Read the model definition and answer for the solid it produces. Units are mm, in the model's axes. A direction names the side the tool comes from. Give positions to 0.01 mm unless a question says otherwise; leave off trailing zeros. Write each loop counter-clockwise with the first axis right and the second up, starting at its lowest first coordinate (ties: lowest second). Pieces come first, ordered by that corner, then holes. Notation, with made-up numbers: M 50.25,32.25 L 87.25,32.25 A23 cw 87.25,54.25 Z; hole C 67,87 d10. An arc over 180 degrees is marked long. Answer as CSV lines item,"result". Start each with the question number.
```python
from build123d import *

# Parameters (mm, degrees)
CROQUIS1_R              = 1.5
SALIENTE_EXTRUIR1_DEPTH = 2.5


with BuildPart() as part:
    # Croquis1 → Saliente-Extruir1 (new body)
    with BuildSketch(Plane(origin=(0, 0, 0), x_dir=(0, 0, -1), z_dir=(1, 0, 0))):
        with BuildLine():
            Line((21.251917537, 86.83352739), (17.00153403, 89.466821912))
            Line((17.00153403, 89.466821912), (18.318181291, 91.592013666))
            Line((18.318181291, 91.592013666), (14.067797783, 94.225308188))
            Line((14.067797783, 94.225308188), (12.751150522, 92.100116434))
            Line((12.751150522, 92.100116434), (4.250383507, 97.366705478))
            Line((4.250383507, 97.366705478), (5.567030768, 99.491897232))
            Line((5.567030768, 99.491897232), (-2.933736246, 104.758486276))
            Line((-2.933736246, 104.758486276), (-4.250383507, 102.633294522))
            Line((-4.250383507, 102.633294522), (-12.751150522, 107.899883566))
            Line((-12.751150522, 107.899883566), (-11.434503261, 110.02507532))
            Line((-11.434503261, 110.02507532), (-15.684886769, 112.658369842))
            Line((-15.684886769, 112.658369842), (-17.00153403, 110.533178088))
            Line((-17.00153403, 110.533178088), (-21.251917537, 113.16647261))
            ThreePointArc((-21.251917537, 113.16647261), (-32.419507908, 26.647274601), (-0.370758332, -54.489427017))
            ThreePointArc((-0.370758332, -54.489427017), (8.867523579, -55.834574652), (11.226722216, -46.801886424))
            ThreePointArc((11.226722216, -46.801886424), (12.220238585, -29.769593029), (20.221051617, -14.700648676))
            ThreePointArc((20.221051617, -14.700648676), (24.926355942, 1.917493015), (17.734708518, 17.620445902))
            ThreePointArc((17.734708518, 17.620445902), (11.831680909, 27.101025049), (10.645879945, 38.206023562))
            ThreePointArc((10.645879945, 38.206023562), (14.782652045, 62.774142971), (21.251917537, 86.83352739))
        make_face()
        with Locations((5, -50)):
            Circle(CROQUIS1_R, mode=Mode.SUBTRACT)
        Circle(CROQUIS1_R, mode=Mode.SUBTRACT)
        with Locations((-5, 30)):
            Circle(CROQUIS1_R, mode=Mode.SUBTRACT)
        with Locations((-5, 70)):
            Circle(CROQUIS1_R, mode=Mode.SUBTRACT)
    extrude(amount=SALIENTE_EXTRUIR1_DEPTH)


solid = part.part
```
1. Find the intervals of material crossed by line 1 (Y direction, x = 1.65, z = 5.5); line 2 (Y direction, x = 0.85, z = 5); line 3 (Z direction, x = 1.6, y = 70), in increasing order. Write a range as [from, to].
2. Find section D-D on z = 19.5. Determine the outline of the cut face in (x, y).
3. Find section A-A on y = 0. Determine the outline of the cut face in (x, z).
4. Find section B-B on x = 1.7. Determine the outline of the cut face in (y, z).
5. Determine the mould class of faces 3 (the face through (2.5, 29, 11)), 4 (the face through (1.232, 27.873, 32.568)), 5 (the face through (1.232, 71.265, 4.194)) for opening direction Y: +Y half, -Y half, draft (parallel to the pull), parting line (faces both ways), or undercut.
6. For faces 1 (the face through (1.2, 62.4, -14.7)), 2 (the face through (1.23, 0.07, 1.5)), determine the directions among +Z, -Z, +X, -X, +Y, -Y from which every point of the face is accessible in a straight line to the end or side of a thin tool.
7. Given pin 1 (2.5 mm diameter, centred on y = -50, z = -5, fed in from +X); pin 2 (1 mm diameter, centred on x = 0.5, z = -7, fed in from -Y); pin 3 (1.5 mm diameter, centred on x = 1.5, z = -15.5, fed in from +Y), each flat-ended and moving along its own axis, determine where each tip first touches the part or whether it passes through.
8. Find section C-C on y = 70. Determine the outline of the cut face in (x, z).
Computed:
1,line 1,"y = [-47.03, 28.59], [31.41, 68.59], [71.41, 103.41]"
1,line 2,"y = [-47.8, 28.5], [31.5, 68.5], [71.5, 103.1]"
1,line 3,"z = [-16.47, 3.5], [6.5, 32.4]"
2,outline,"M 0,-20.89 L 2.5,-20.89 L 2.5,112.08 L 0,112.08 Z"
3,outline,"M 0,-25 L 2.5,-25 L 2.5,-1.5 L 0,-1.5 Z; M 0,1.5 L 2.5,1.5 L 2.5,26.97 L 0,26.97 Z"
4,outline,"M -54.49,0.37 A7 ccw -46.8,-11.23 A40 cw -14.7,-20.22 A25 ccw 17.62,-17.73 A25 cw 38.21,-10.65 A260 cw 86.83,-21.25 L 89.47,-17 L 91.59,-18.32 L 94.23,-14.07 L 92.1,-12.75 L 97.37,-4.25 L 99.49,-5.57 L 104.76,2.93 L 102.63,4.25 L 107.9,12.75 L 110.03,11.43 L 112.66,15.68 L 110.53,17 L 113.17,21.25 A174.75 ccw Z; hole C -50,-5 d3; hole C 0,0 d3; hole C 30,5 d3; hole C 70,5 d3"
5,face 3,"draft"
5,face 4,"parting line"
5,face 5,"undercut"
6,face 1,"-Z, +X, -X"
6,face 2,"+X, -X"
7,pin 1,"passes through"
7,pin 2,"stops at y = -56.84"
7,pin 3,"stops at y = 93.8"
8,outline,"M 0,-16.47 L 2.5,-16.47 L 2.5,3.5 L 0,3.5 Z; M 0,6.5 L 2.5,6.5 L 2.5,32.4 L 0,32.4 Z"
